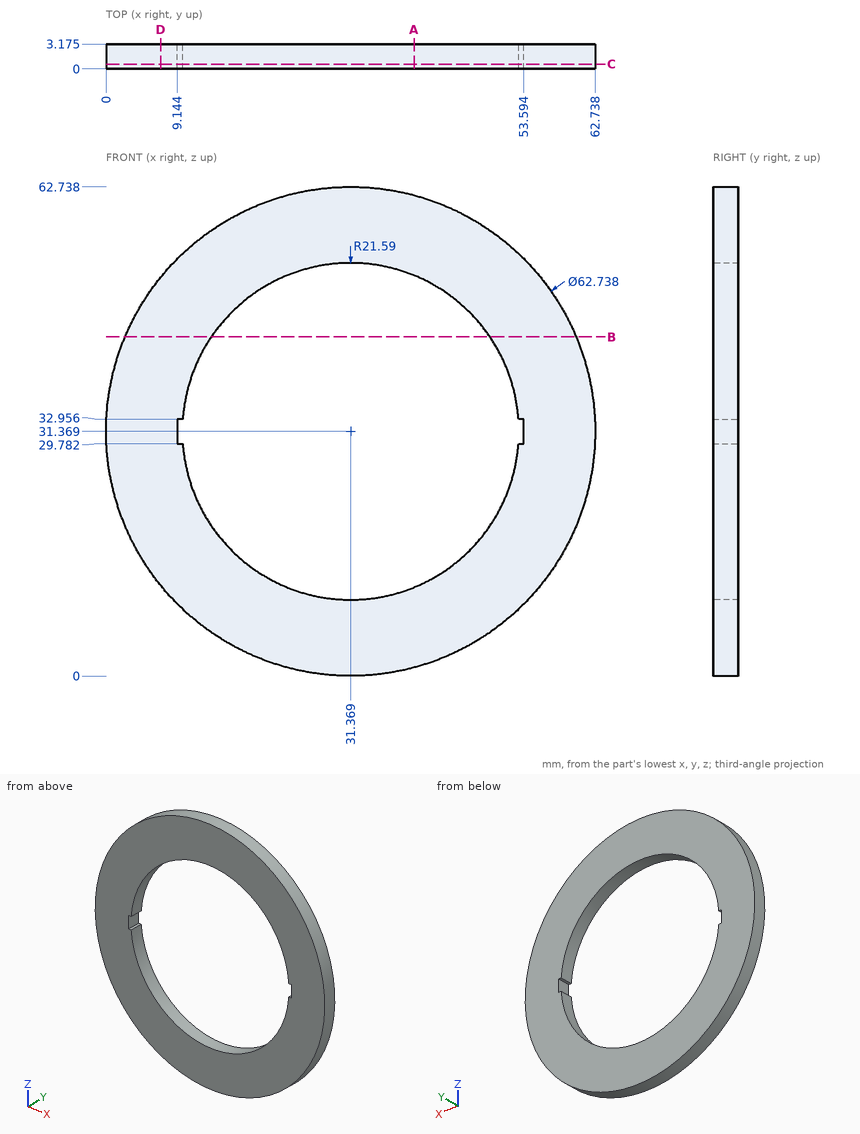
Answer from the drawing. Dimensions are ordinates in mm from the lowest x, y and z of the part. Give positions to 0.01 mm unless a question says otherwise; leave off trailing zeros. Loops run counter-clockwise (first coordinate to the right, second up) from the corner with the lowest first, then second, coordinate; pieces in that order, holes last.
Item 1: Each of these flat-tipped pins is pushed along its axis until it touches: pin 1 Ø1 at (y, z) = (1.5, 31.5) entering from +X; pin 2 Ø1 at (x, y) = (19.5, 1) entering from -Z; pin 3 Ø0.8 at (x, y) = (53.5, 2) entering from +Z; pin 4 Ø10 at (x, z) = (12.5, 30.5) entering from +Y (1 decimal). Where does it stop, or does it pass through?
Item 2: The part is cut by section C-C (y = 0.6). Write down the section's boundary in (x, z) (1 decimal).
Item 3: Find the intervals of material crossed by line 1 along X through (y, z) = (1.8, 47) (1 decimal); line 2 along X through (y, z) = (2.2, 41) (1 decimal); line 3 along Z through (x, y) = (9.5, 2.85) (1 decimal), in increasing order.
Item 4: The part is cut by section B-B (z = 43.5). Write down the section's boundary in (x, y) (1 decimal).
Item 5: The part is cut by section D-D (x = 7). Write down the section's boundary in (y, z) (1 decimal).
Item 6: The part is cut by section A-A (x = 39.5). Write down the section's boundary in (y, z) (1 decimal).
Taken from the geometry:
1. pin 1: stops at x = 62.74
1. pin 2: stops at z = 2.13
1. pin 3: stops at z = 53.99
1. pin 4: stops at y = 3.2
2. outline: circle Ø62.7 at (31.4, 31.4); hole (9.1, 29.8) - (9.8, 29.8) arc R21.6 ccw to (52.9, 29.8) - (53.6, 29.8) - (53.6, 33) - (52.9, 33) arc R21.6 ccw to (9.8, 33) - (9.1, 33) - close
3. line 1: x = 4.2 to 16.5, 46.3 to 58.6
3. line 2: x = 1.5 to 12, 50.7 to 61.2
3. line 3: z = 8.9 to 29.8, 33 to 53.9
4. outline: (2.4, 0) - (13.5, 0) - (13.5, 3.2) - (2.4, 3.2) - close; (49.2, 0) - (60.3, 0) - (60.3, 3.2) - (49.2, 3.2) - close
5. outline: (0, 11.6) - (3.2, 11.6) - (3.2, 51.1) - (0, 51.1) - close
6. outline: (0, 1.1) - (3.2, 1.1) - (3.2, 11.4) - (0, 11.4) - close; (0, 51.4) - (3.2, 51.4) - (3.2, 61.7) - (0, 61.7) - close
